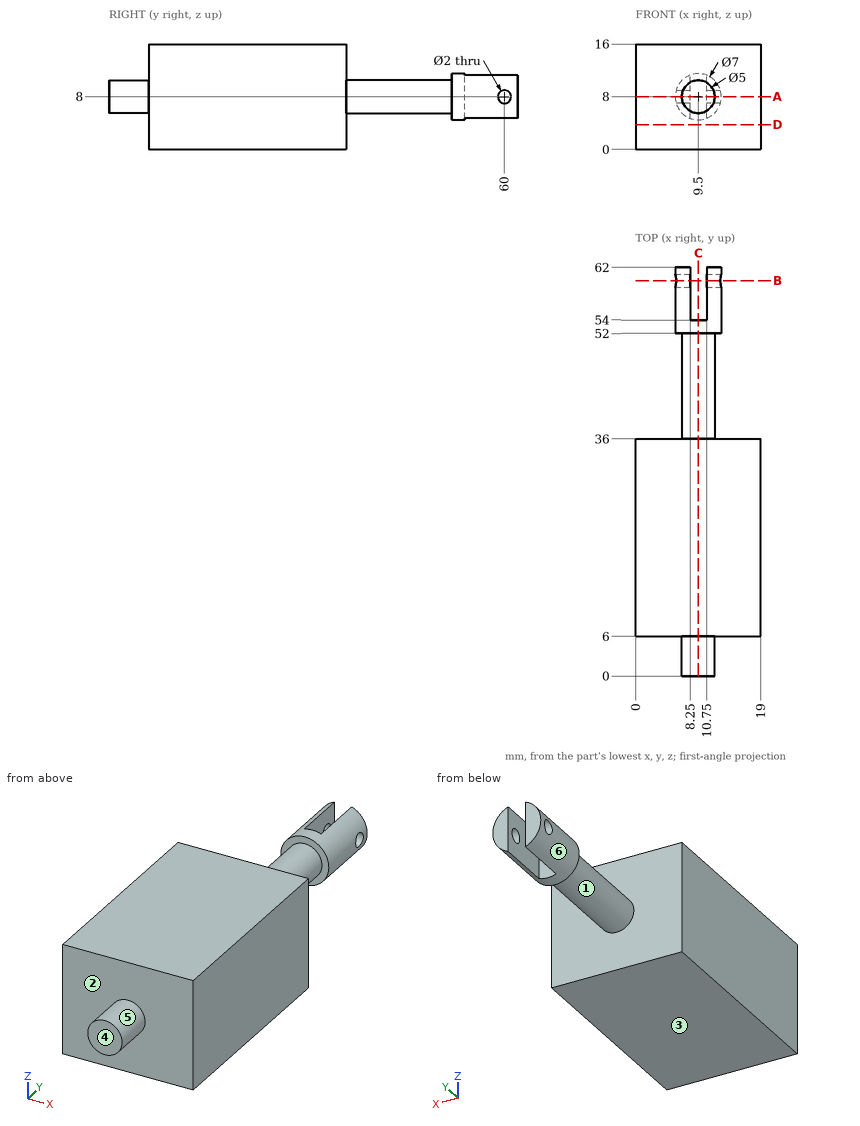
Print and shaded views of the part. All mm, measured from the part's lowest x, y and z. A direction names the side the tool comes from. Coordinates: 2 decimals unless noted, no trailing zeros. Order: outer loops, then holes, each group sorted by start corner. A loop starts at its lowest first (then second) coordinate and runs counter-clockwise, first axis right, second up. Notation, with made-up numbers: (-5, 45) -> (30, 45) arc R33 ccw to (30, 75) -> close; hole circle Ø4 at (11.5, -29). An arc over 180 degrees is marked (long way). Use one line per item in the form item = value. Start each with the question number.
1) Band-saw the part on B-B on y = 60. Give the cut face in (x, z).
2) Pull direction Y, two halves, no side cores. Call the marked faces 1, 2 and 3: +Y half, -Y half, draft (parallel to the pull), parting line (faces both ways), or undercut.
3) Drill centre lines: L1, parallel to Y at x = 12.2, z = 8; L2, parallel to Y at x = 11.25, z = 5; L3, parallel to Y at x = 7.4, z = 8. Where is each one in solid material? Low to high. Write a range as [from, to].
4) Band-saw the part on D-D on z = 3.75. Give the cut face in (x, y).
5) Band-saw the part on A-A on z = 8. Give the cut face in (x, y), then the cut area to 3 significant figures.
6) Tool access for the marked faces 4, 5 and 6: list every direction of +Z, -Z, +X, -X, +Y, -Y with a clear straight run to the whole face (end or side of a thin tool).
7) Band-saw the part on C-C on x = 9.5. Give the cut face in (y, z).
8) Drop flat-ended pins along their axis: pin 1 (0.8 mm diameter, centred on x = 9.5, z = 8.5, fed in from +Y); pin 2 (8 mm diameter, centred on x = 8.5, z = 8, fed in from +Y); pin 3 (5 mm diameter, centred on x = 3, y = 53.5, fed in from +Z); pin 4 (3.5 mm diameter, centred on y = 58.5, z = 9.5, fed in from +X). Give the stop position or say it passes through.
Entries:
q1.outline = (6.15, 7) arc R3.5 ccw to (8.25, 4.73) -> (8.25, 7) -> close; (6.15, 9) -> (8.25, 9) -> (8.25, 11.27) arc R3.5 ccw to start; (10.75, 4.73) arc R3.5 ccw to (12.85, 7) -> (10.75, 7) -> close; (10.75, 9) -> (12.85, 9) arc R3.5 ccw to (10.75, 11.27) -> close
q2.face_1 = undercut
q2.face_2 = -Y half
q2.face_3 = draft
q3.L1 = [6, 36], [52, 59], [61, 62]
q3.L2 = [6, 36], [52, 62]
q3.L3 = [0, 59], [61, 62]
q4.outline = (0, 6) -> (19, 6) -> (19, 36) -> (0, 36) -> close
q5.outline = (0, 6) -> (7, 6) -> (7, 0) -> (12, 0) -> (12, 6) -> (19, 6) -> (19, 36) -> (12, 36) -> (12, 52) -> (13, 52) -> (13, 59) -> (10.75, 59) -> (10.75, 54) -> (8.25, 54) -> (8.25, 59) -> (6, 59) -> (6, 52) -> (7, 52) -> (7, 36) -> (0, 36) -> close; (6, 61) -> (8.25, 61) -> (8.25, 62) -> (6, 62) -> close; (10.75, 61) -> (13, 61) -> (13, 62) -> (10.75, 62) -> close
q5.area = 721 mm2
q6.face_4 = +Z, -Z, +X, -X, -Y
q6.face_5 = -Y
q6.face_6 = +Y
q7.outline = (0, 5.5) -> (6, 5.5) -> (6, 0) -> (36, 0) -> (36, 5.5) -> (52, 5.5) -> (52, 4.5) -> (54, 4.5) -> (54, 11.5) -> (52, 11.5) -> (52, 10.5) -> (36, 10.5) -> (36, 16) -> (6, 16) -> (6, 10.5) -> (0, 10.5) -> close
q8.pin_1 = 54
q8.pin_2 = 62
q8.pin_3 = through
q8.pin_4 = 13
